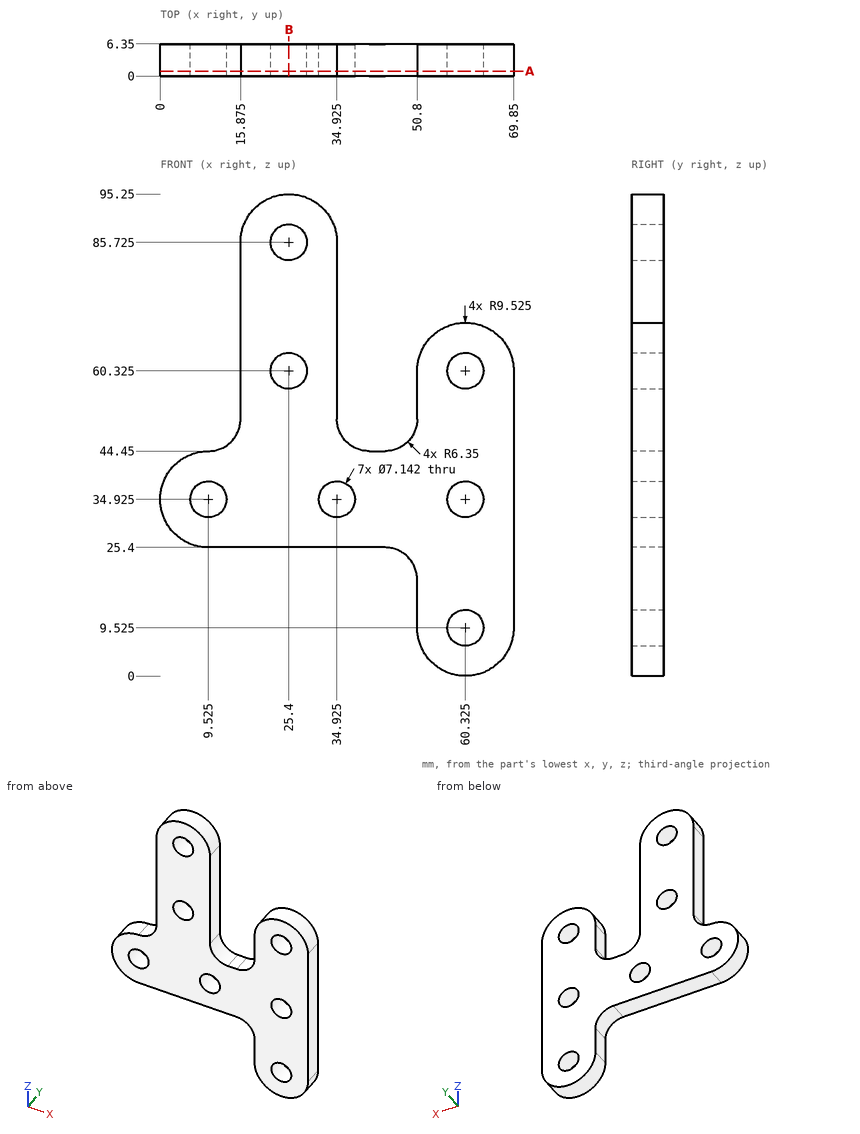
For this review, use the dimensioned drawing (mm, ordinates from the lowest corner) and the shaded views. Round coordinates to 2 decimals unless told otherwise and drop trailing zeros. Order: outer loops, then holes, each group sorted by start corner. A loop starts at its lowest first (then second) coordinate and runs counter-clockwise, first axis right, second up.
1) For L1, parallel to Z at x = 60, y = 1.5 (1 decimal); L2, parallel to Z at x = 22.5, y = 1 (1 decimal); L3, parallel to Z at x = 43.5, y = 0.75, list the stretches that pass through material, from the lowest coordinate up.
The answers:
L1: z = 0 to 6, 13.1 to 31.4, 38.5 to 56.8, 63.9 to 69.8
L2: z = 25.4 to 58.2, 62.4 to 83.6, 87.8 to 94.8
L3: z = 25.4 to 44.45
2) Clearance check with flat-ended pins moving along their axes: pin 1 Ø3 at (y, z) = (1.5, 71.5) entering from -X (1 decimal); pin 2 Ø1.9 at (y, z) = (2, 16) entering from -X; pin 3 Ø4.5 at (x, z) = (34.925, 34.925) entering from +Y; pin 4 Ø8 at (x, z) = (25.4, 60.325) entering from +Y. State where each tip first meets the part, or that it passes through.
The answers:
pin 1: stops at x = 15.9
pin 2: stops at x = 50.8
pin 3: passes through
pin 4: stops at y = 6.35
3) Consider section B-B (x = 25.4). State the section outline as (y, z) points.
The answers:
outline: (0, 25.4) - (6.35, 25.4) - (6.35, 56.75) - (0, 56.75) - close; (0, 63.9) - (6.35, 63.9) - (6.35, 82.15) - (0, 82.15) - close; (0, 89.3) - (6.35, 89.3) - (6.35, 95.25) - (0, 95.25) - close
4) Consider section A-A (y = 1). Count the separate pieces of the cut face and the enclosed holes in it, plus the area to 3 significant figures.
The answers:
separate pieces: 1
enclosed holes: 7
area: 2,860 mm2
